Job drawing, mm, ordinate dimensions from the low corner. One solid piece. Coordinates: 2 decimals unless noted, no trailing zeros. Order: outer loops, then holes, each group sorted by start corner. A loop starts at its lowest first (then second) coordinate and runs counter-clockwise, first axis right, second up. Notation, with made-up numbers: (27, -39.5) - (82, -39.5) arc R10 ccw to (82, -33.5) - close; hole circle Ø8 at (14.5, 54.5). An arc over 180 degrees is marked (long way). Return JSON: item names as keys, results as strings.
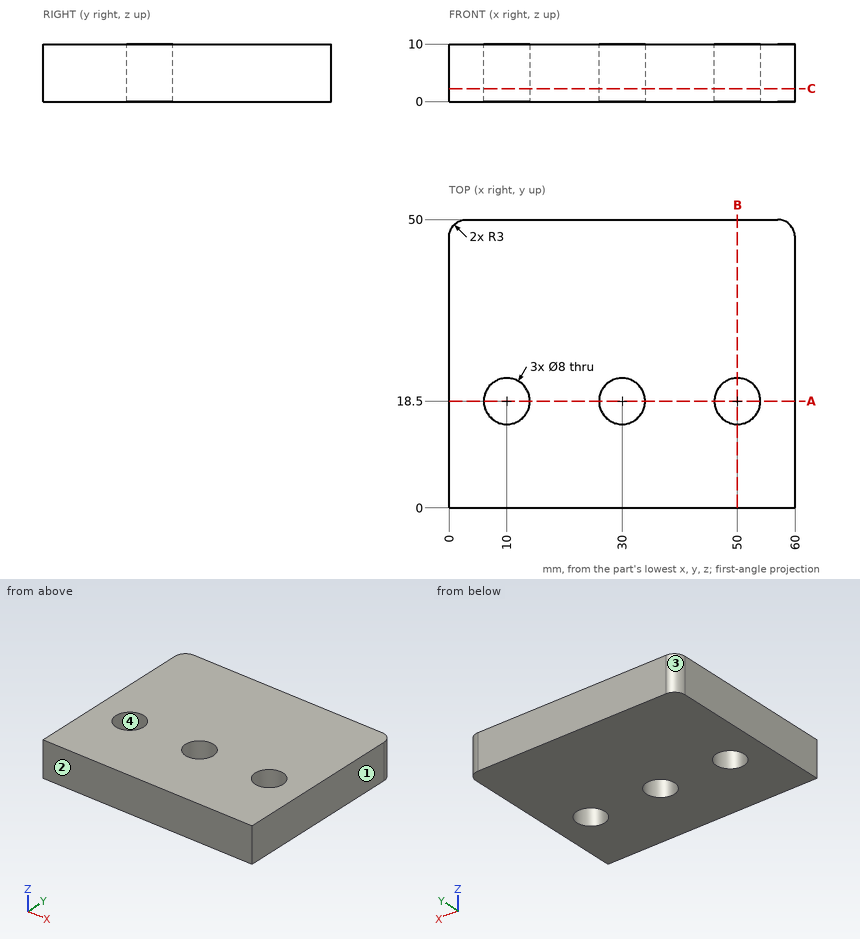
1. Mould opens along X. For the marked faces 1, 2, 3 and 4 say: pulls with the +X half, pulls with the -X half, needs draft (parallel to the pull), parting line crosses it, or undercut.
Check values:
{"face 1": "pulls with the +X half", "face 2": "needs draft", "face 3": "pulls with the -X half", "face 4": "undercut"}
2. Probe L1, parallel to Y at x = 10, z = 5; L2, parallel to Y at x = 49, z = 2.75. List the from-to ranges inside material, lowest first.
Check values:
{"L1": "0 to 14.5, 22.5 to 50", "L2": "0 to 14.63, 22.37 to 50"}
3. Cut at B-B on x = 50. Give the cut face in (y, z).
Check values:
{"outline": "(0, 0) - (14.5, 0) - (14.5, 10) - (0, 10) - close; (22.5, 0) - (50, 0) - (50, 10) - (22.5, 10) - close"}
4. Cut at A-A on y = 18.5. Give the cut face in (x, z), plus the area to 3 significant figures.
Check values:
{"outline": "(0, 0) - (6, 0) - (6, 10) - (0, 10) - close; (14, 0) - (26, 0) - (26, 10) - (14, 10) - close; (34, 0) - (46, 0) - (46, 10) - (34, 10) - close; (54, 0) - (60, 0) - (60, 10) - (54, 10) - close", "area": "360 mm²"}
5. Cut at C-C on z = 2.25. Give the cut face in (x, y).
Check values:
{"outline": "(0, 0) - (60, 0) - (60, 47) arc R3 ccw to (57, 50) - (3, 50) arc R3 ccw to (0, 47) - close; hole circle Ø8 at (10, 18.5); hole circle Ø8 at (30, 18.5); hole circle Ø8 at (50, 18.5)"}
